from build123d import *

# Parameters (mm, degrees)
SKETCH1_R           = 1.25
BOSS_EXTRUDE9_DEPTH = 5
CUT_EXTRUDE1_DEPTH  = 10


with BuildPart() as part:
    # Sketch1 → Boss-Extrude9 (new body)
    with BuildSketch(Plane(origin=(0, 0, 0), x_dir=(1, 0, 0), z_dir=(0, 1, 0))):
        with BuildLine():
            Line((23.600035939, 26.479209334), (48.489298853, 3.430633728))
            ThreePointArc((48.489298853, 3.430633728), (53.57304499, 11.525457211), (59.99370362, 18.606826058))
            ThreePointArc((59.99370362, 18.606826058), (122.945468319, 87.076417595), (191.415059857, 150.028182295))
            ThreePointArc((191.415059857, 150.028182295), (191.413333308, 170.020159366), (171.421356237, 170.021885915))
            ThreePointArc((171.421356237, 170.021885915), (108.469591538, 101.552294377), (40, 38.600529677))
            ThreePointArc((40, 38.600529677), (32.372407148, 31.765435558), (23.600035939, 26.479209334))
        make_face()
        with Locations(Location((41.868272016, 31.782510193, 0), (0, 0, 270))):
            Circle(SKETCH1_R, mode=Mode.SUBTRACT)
        with Locations(Location((36.918524548, 26.832762725, 0), (0, 0, 270))):
            Circle(SKETCH1_R, mode=Mode.SUBTRACT)
        with Locations(Location((48.232233047, 15.519054226, 0), (0, 0, 270))):
            Circle(SKETCH1_R, mode=Mode.SUBTRACT)
        with Locations(Location((53.181980515, 20.468801694, 0), (0, 0, 270))):
            Circle(SKETCH1_R, mode=Mode.SUBTRACT)
        with BuildLine():
            Line((187.351349634, 164.261119417), (185.65429336, 165.958175692))
            Line((185.65429336, 165.958175692), (182.118759454, 162.422641786))
            ThreePointArc((182.118759454, 162.422641786), (181.416481349, 162.523307407), (180.714203245, 162.422641786))
            Line((180.714203245, 162.422641786), (177.178669339, 165.958175692))
            Line((177.178669339, 165.958175692), (175.481613064, 164.261119417))
            Line((175.481613064, 164.261119417), (179.01714697, 160.725585511))
            ThreePointArc((179.01714697, 160.725585511), (178.916481349, 160.023307407), (179.01714697, 159.321029302))
            Line((179.01714697, 159.321029302), (175.481613064, 155.785495396))
            Line((175.481613064, 155.785495396), (177.178669339, 154.088439122))
            Line((177.178669339, 154.088439122), (180.714203245, 157.623973027))
            ThreePointArc((180.714203245, 157.623973027), (181.416481349, 157.523307407), (182.118759454, 157.623973027))
            Line((182.118759454, 157.623973027), (185.65429336, 154.088439122))
            Line((185.65429336, 154.088439122), (187.351349634, 155.785495396))
            Line((187.351349634, 155.785495396), (183.815815728, 159.321029302))
            ThreePointArc((183.815815728, 159.321029302), (183.916481349, 160.023307407), (183.815815728, 160.725585511))
            Line((183.815815728, 160.725585511), (187.351349634, 164.261119417))
        make_face(mode=Mode.SUBTRACT)
        with BuildLine():
            Line((47.878679656, 29.307636459), (50.707106781, 26.479209334))
            ThreePointArc((50.707106781, 26.479209334), (51, 25.772102553), (50.707106781, 25.064995772))
            Line((50.707106781, 25.064995772), (43.636038969, 17.99392796))
            ThreePointArc((43.636038969, 17.99392796), (42.928932188, 17.701034741), (42.221825407, 17.99392796))
            Line((42.221825407, 17.99392796), (39.393398282, 20.822355084))
            ThreePointArc((39.393398282, 20.822355084), (39.100505063, 21.529461866), (39.393398282, 22.236568647))
            Line((39.393398282, 22.236568647), (46.464466094, 29.307636459))
            ThreePointArc((46.464466094, 29.307636459), (47.171572875, 29.600529677), (47.878679656, 29.307636459))
        make_face(mode=Mode.SUBTRACT)
    extrude(amount=BOSS_EXTRUDE9_DEPTH)

    # Sketch3 → Cut-Extrude1 (cut)
    with BuildSketch(Plane(origin=(0, 5, 0), x_dir=(1, 0, 0), z_dir=(0, 1, 0))):
        Polygon((53.506506714, 32.107245232), (54.710738681, 43.14334784), (58.999320763, 41.803165939), (62.394448245, 47.431929922), (68.830431901, 47.431929922), (68.830750881, 40.995946275), (63.202155174, 37.600539824), (64.542549624, 33.312024169), align=None)
        Polygon((81.21135591, 59.813467571), (90.79476364, 75.829325012), (99.384762751, 77.987775145), (97.226738359, 69.397669067), align=None)
        Polygon((118.033043481, 96.636980145), (117.02456542, 101.302497895), (106.053446407, 88.187597005), (110.557637166, 89.161203324), (109.584254085, 84.656964316), (122.698611208, 95.628733318), align=None)
        Polygon((130.769320539, 109.373888454), (134.174820431, 123.118631106), (139.902949275, 121.699387207), (145.650358709, 133.585330855), (155.989652523, 134.59547044), (154.980025376, 124.256126574), (143.094366596, 118.508128056), (144.513894391, 112.780069559), align=None)
        Polygon((163.041484482, 141.647651911), (159.946738621, 149.458162099), (163.041484482, 150.684388263), (169.998774874, 150.684388263), (169.246288288, 147.852763247), (172.077876006, 148.605390173), (172.078220823, 141.64809979), (170.852148043, 138.553293158), align=None)
    extrude(amount=-CUT_EXTRUDE1_DEPTH, mode=Mode.SUBTRACT)


solid = part.part
Verification items for the finished model (mm, model axes). Give positions to 0.01 mm unless a question says otherwise; leave off trailing zeros. Loops run counter-clockwise (first coordinate to the right, second up) from the corner with the lowest first, then second, coordinate; pieces in that order, holes last.
1. Material ranges on probe 1 along Z at (x, y) = (187, 4); probe 2 along Z at (x, y) = (185.5, 0.9); probe 3 along Z at (x, y) = (121.5, 3), recorded low to high.
Derived:
probe 1: z = -173.01 to -164.61, -163.91 to -156.14, -155.43 to -146.28
probe 2: z = -173.56 to -165.8, -162.41 to -157.64, -154.24 to -145
probe 3: z = -114.8 to -95.89, -94.63 to -85.63
2. Cross-section at C-C on y = 4.25. Count the separate pieces of the cut face and the enclosed holes in it, and give its area (3 significant figures).
Derived:
separate pieces: 1
enclosed holes: 11
area: 4,290 mm2
3. Go/stop test with flat-tipped pins: P1, Ø2.5, axis at y = 2, z = -44.5, coming from the -X side; P2, Ø1, axis at x = 104, y = 1.5, coming from the -Z side; P3, Ø2.5, axis at y = 3, z = -146, coming from the -X side; P4, Ø3, axis at x = 36.92, z = -26.83, coming from the +Y side. Record where each tip stops, or that it passes through.
Derived:
P1: stops at x = 45.47
P2: stops at z = -97.6
P3: stops at x = 149.41
P4: stops at y = 5
4. Cross-section at B-B on x = 151. Record the cut outline in (y, z), and give its area (3 significant figures).
Derived:
outline: (0, -146.53) - (5, -146.53) - (5, -134.11) - (0, -134.11) - close; (0, -122.33) - (5, -122.33) - (5, -114.16) - (0, -114.16) - close
area: 103 mm2
5. Cross-section at A-A on z = -92. Record the cut outline in (x, y), and give its area (3 significant figures).
Derived:
outline: (98.8, 0) - (109.24, 0) - (109.24, 5) - (98.8, 5) - close; (118.36, 0) - (127.9, 0) - (127.9, 5) - (118.36, 5) - close
area: 99.9 mm2
6. Cross-section at D-D on x = 77.5. Record the cut outline in (y, z).
Derived:
outline: (0, -71.76) - (5, -71.76) - (5, -38.83) - (0, -38.83) - close
7. Release check for a two-part mould opening along X. For faces 1 (the flat face through (120.398, 2.535, -96.126)), 2 (the cylindrical face through (53.492, 2.465, -11.419)), 3 (the flat face through (109, 5, -83)) record: +X half, -X half, draft (parallel to the pull), parting line (faces both ways), or undercut.
Derived:
face 1: undercut
face 2: +X half
face 3: draft
